Study the drawing (mm; zero at the part's minimum x, y, z) and answer. Coordinates: 2 decimals unless noted, no trailing zeros. Loops run counter-clockwise (first coordinate to the right, second up) from the corner with the lowest first, then second, coordinate; pieces in that order, holes last. Notation, with made-up numbers: (-34.5, 31) - (3.5, 31) arc R29 ccw to (3.5, 59) - close; hole circle Ø5 at (-25, -25.5). An arc over 180 degrees is marked (long way). Write each question's results on one line, items separated by ' | '. Start each with the question number.
(1) Given pin 1 Ø5 at (x, z) = (7.575, 7.575) entering from -Y; pin 2 Ø8 at (x, z) = (26.5, 68.5) entering from -Y; pin 3 Ø1.5 at (y, z) = (1, 81) entering from -X, each flat-ended and moving along its own axis, determine where each tip first touches the part or whether it passes through.
(2) Consider line 1 (Z direction, x = 5, y = 3.2); line 2 (Y direction, x = 26, z = 47); line 3 (Z direction, x = 10, y = 4.6). Determine where each line is inside the solid, lowest interval first. Write a range as from..to.
(3) Find section B-B on x = 50. Determine the outline of the cut face in (y, z).
(4) Determine the mould class of the marked faces 1 and 2 for opening direction X: released by +X, released by -X, zero draft, split by the parting line, or undercut.
(5) Find section C-C on y = 2. Determine the outline of the cut face in (x, z).
(6) Find section A-A on z = 50. Determine the outline of the cut face in (x, y), then the cut area to 3 significant figures.
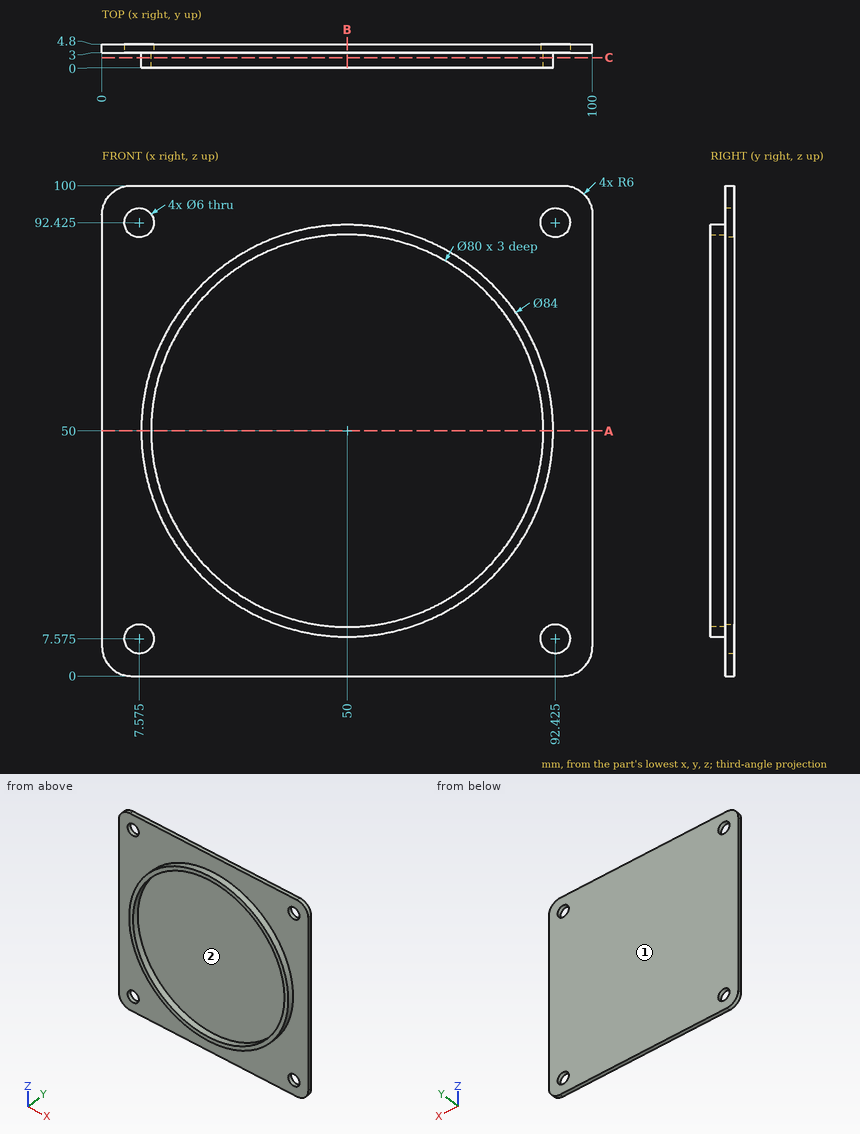
Values:
1) pin 1: passes through | pin 2: stops at y = 3 | pin 3: stops at x = 20.86
2) line 1: z = 0.08..6.04, 9.11..90.89, 93.96..99.92 | line 2: y = 3..4.8 | line 3: z = 0..5.81, 9.34..90.66, 94.19..100
3) outline: (0, 8) - (3, 8) - (3, 0) - (4.8, 0) - (4.8, 100) - (3, 100) - (3, 92) - (0, 92) - (0, 90) - (3, 90) - (3, 10) - (0, 10) - close
4) face 1: zero draft | face 2: undercut
5) outline: circle Ø84 at (50, 50); hole circle Ø80 at (50, 50)
6) outline: (0, 3) - (8, 3) - (8, 0) - (10, 0) - (10, 3) - (90, 3) - (90, 0) - (92, 0) - (92, 3) - (100, 3) - (100, 4.8) - (0, 4.8) - close | area: 192 mm²
